Input: part model. Units: mm. Frame: model coordinates. Face numbers are marked on the shaded views. A direction names the side the tool comes from. Round coordinates to 2 decimals unless told otherwise and drop trailing zeros. Write each loop counter-clockwise with the first axis right and the second up, starting at its lowest first coordinate (ties: lowest second). Pieces come first, ordered by that corner, then holes. Notation, with made-up numbers: M -22.75,64.5 L 9.25,64.5 A11 cw 9.25,78.5 Z; hole C -2.5,48 d2. An arc over 180 degrees is marked long. Use one line per item in the form item = value. Start each with the question number.
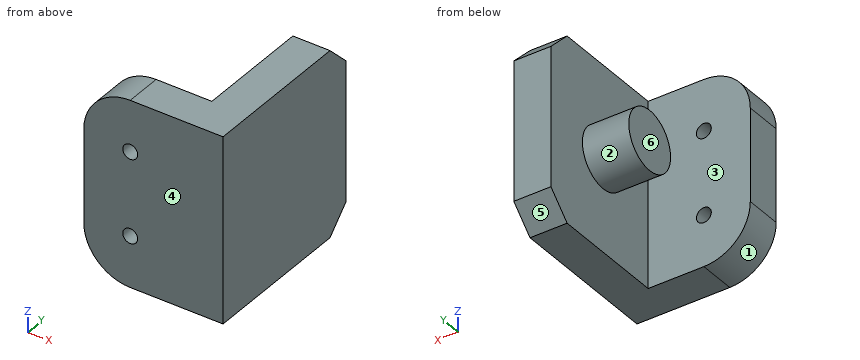
```python
from build123d import *

# Parameters (mm, degrees)
CROQUIS1_W              = 4
CROQUIS1_H              = 30
CROQUIS1_H_2            = 8
SALIENTE_EXTRUIR1_DEPTH = 20
CROQUIS2_R              = 6.44
SALIENTE_EXTRUIR2_DEPTH = 10
CHAFL_N1_SIZE           = 5
REDONDEO1_R             = 10
CROQUIS3_R              = 1.6
CORTAR_EXTRUIR1_DEPTH   = 10


with BuildPart() as part:
    # Croquis1 → Saliente-Extruir1 (new, symmetric)
    with BuildSketch(Plane.XY):
        with Locations((-2, 19)):
            Rectangle(CROQUIS1_W, CROQUIS1_H)
        with Locations((2, 19)):
            Rectangle(CROQUIS1_W, CROQUIS1_H)
        Polygon((0, -4), (0, 4), (-4, 4), (-26, 4), (-26, -4), align=None)
        with Locations((2, 0)):
            Rectangle(CROQUIS1_W, CROQUIS1_H_2)
    extrude(amount=SALIENTE_EXTRUIR1_DEPTH, both=True)

    # Croquis2 → Saliente-Extruir2 (add)
    with BuildSketch(Plane.ZY.offset(4)):
        with Locations(Location((0, 17.85, 0), (0, 0, 270))):
            Circle(CROQUIS2_R)
    extrude(amount=SALIENTE_EXTRUIR2_DEPTH)

    # Chaflán1
    chafl_n1_edges = [part.edges().sort_by_distance(p)[0] for p in [
        (0, 34, 20),
        (0, 34, -20),
    ]]
    chamfer(chafl_n1_edges, length=CHAFL_N1_SIZE)

    # Redondeo1
    redondeo1_edges = [part.edges().sort_by_distance(p)[0] for p in [
        (-26, 0, 20),
        (-26, 0, -20),
    ]]
    fillet(redondeo1_edges, radius=REDONDEO1_R)

    # Croquis3 → Cortar-Extruir1 (cut)
    with BuildSketch(Plane.XZ.offset(4)):
        with Locations((-16, 9)):
            Circle(CROQUIS3_R)
        with Locations(Location((-16, -9, 0), (0, 0, 180))):
            Circle(CROQUIS3_R)
    extrude(amount=-CORTAR_EXTRUIR1_DEPTH, mode=Mode.SUBTRACT)


solid = part.part
```
Item 1: Cut plane B-B (x = -1). Output: boundary loops of the cut face in (y, z), plus the area to 4 significant figures.
Item 2: First-contact query: pin 1 (3.5 mm diameter, centred on x = -16, z = -9, fed in from +Y); pin 2 (17.5 mm diameter, centred on x = -15, z = -8, fed in from +Y); pin 3 (3 mm diameter, centred on y = 23, z = 15, fed in from -X). Flat tips, straight axial feed; report the tip coordinate or a pass-through.
Item 3: Ray query, line 1 (Z direction, x = -16, y = -2); line 2 (X direction, y = -1, z = -9); line 3 (X direction, y = 4.5, z = -14). Return the intervals inside material, ascending. Write a range as from..to.
Item 4: Cut plane D-D (z = 0). Output: boundary loops of the cut face in (x, y), plus the area to 3 significant figures.
Item 5: Cut plane C-C (y = 17.85). Output: boundary loops of the cut face in (x, z).
Item 6: Draft query along Y for the marked faces 1, 2, 3 and 4. Return one class per face: +Y half, -Y half, draft (parallel to the pull), parting line (faces both ways), or undercut.
Item 7: Cut plane A-A (z = -9). Output: boundary loops of the cut face in (x, y).
Item 8: Reachability of the marked faces 5 and 6 from +Z, -Z, +X, -X, +Y, -Y: full face, straight path, thin tool, end or side. Return the list, or none.
Final values:
q1.outline = M -4,-20 L 29,-20 L 34,-15 L 34,15 L 29,20 L -4,20 Z
q1.area = 1,495 mm^2
q2.pin_1 = 4
q2.pin_2 = 24.29
q2.pin_3 = -4
q3.line_1 = -20..-10.6, -7.4..7.4, 10.6..20
q3.line_2 = -26..-17.6, -14.4..4
q3.line_3 = -4..4
q4.outline = M -26,-4 L 4,-4 L 4,34 L -4,34 L -4,24.29 L -14,24.29 L -14,11.41 L -4,11.41 L -4,4 L -26,4 Z
q4.area = 609 mm^2
q5.outline = M -14,-6.44 L -4,-6.44 L -4,-20 L 4,-20 L 4,20 L -4,20 L -4,6.44 L -14,6.44 Z
q6.face_1 = draft
q6.face_2 = undercut
q6.face_3 = undercut
q6.face_4 = -Y half
q7.outline = M -26,-4 L -17.6,-4 L -17.6,4 L -26,4 Z; M -14.4,-4 L 4,-4 L 4,34 L -4,34 L -4,4 L -14.4,4 Z
q8.face_5 = -Z, +X, -X, +Y
q8.face_6 = +Z, -Z, -X, +Y
